Input: part model. Units: mm. Frame: model coordinates. A direction names the side the tool comes from. Coordinates: 2 decimals unless noted, no trailing zeros. Loops run counter-clockwise (first coordinate to the right, second up) from the corner with the lowest first, then second, coordinate; pieces in that order, holes last. Notation, with made-up numbers: (17, 35) - (74, 35) arc R30 ccw to (74, 68) - close; hole circle Ø2 at (21.25, 17). An arc over 180 degrees is marked (long way). Answer as CSV lines item,"result". Start each with the question number.
```python
from build123d import *

# Parameters (mm, degrees)
SM_START               = -47.5
SM_BASE_FLANGE_1_DEPTH = 95
CUT_EXTRUDE_1_DEPTH    = 278.911623222
FILLET_1_R             = 10


# Read off the part's stored shape, not the designer's step: 基体-法兰1
with BuildPart() as part:
    # 基体-法兰1 outline → 基体-法兰1 (new body)
    with BuildSketch(Plane(origin=(0, 0, 0), x_dir=(0, 0, -1), z_dir=(1, 0, 0)).offset(SM_START)):
        with BuildLine():
            Line((20.994484106, 56.207042593), (-70.293536893, 90.304992202))
            Line((-70.293536893, 90.304992202), (-73.092801441, 82.810719856))
            Line((-73.092801441, 82.810719856), (18.195219559, 48.712770248))
            ThreePointArc((18.195219559, 48.712770248), (51.999935218, -0.082081346), (18.041344088, -48.769969279))
            Line((18.041344088, -48.769969279), (-51.521246849, -74.503072197))
            ThreePointArc((-51.521246849, -74.503072197), (-52.886976122, -74.874788174), (-54.296838247, -75))
            Line((-54.296838247, -75), (-212, -75))
            Line((-212, -75), (-212, -83))
            Line((-212, -83), (-54.296838247, -83))
            ThreePointArc((-54.296838247, -83), (-51.477113996, -82.749576348), (-48.74565545, -82.006144394))
            Line((-48.74565545, -82.006144394), (20.816935486, -56.273041476))
            ThreePointArc((20.816935486, -56.273041476), (59.999925251, -0.094709246), (20.994484106, 56.207042593))
        make_face()
    extrude(amount=SM_BASE_FLANGE_1_DEPTH)

    # 草图6 → 切除-拉伸1 (cut, through all)
    with BuildSketch(Plane.XZ.offset(83)):
        with BuildLine():
            Line((-25, 162), (-25, 212))
            Line((-25, 212), (25, 212))
            Line((25, 212), (25, 162))
            ThreePointArc((25, 162), (0, 137), (-25, 162))
        make_face()
    extrude(amount=-CUT_EXTRUDE_1_DEPTH, mode=Mode.SUBTRACT)

    # 圆角1
    fillet_1_edges = [part.edges().sort_by_distance(p)[0] for p in [
        (-25, -79, 212),
        (25, -79, 212),
    ]]
    fillet(fillet_1_edges, radius=FILLET_1_R)


solid = part.part
```
Item 1: Draft query along Y for faces 1 (the cylindrical face through (-0.66, -1.12, -59.99)), 2 (the cylindrical face through (0.55, -79.056, 137.006)), 3 (the flat face through (-0.665, -61.456, 16.253)), 4 (the flat face through (-0.665, 73.017, 24.011)). Return one class per face: pulls with the +Y half, pulls with the -Y half, needs draft (parallel to the pull), parting line crosses it, or undercut.
Item 2: Set-up query: faces 5 (the cylindrical face through (-28.01, -78.94, 209.15)), 6 (the flat face through (-0.66, 66, 28.09)), 7 (the flat face through (47.5, -67, 26)). Return all of +Z, -Z, +X, -X, +Y, -Y with unobstructed straight access to the full face (end or side cutting, diameter ignored); none if empty.
Item 3: Section query B-B, the plane z = 119. Output: boundary loops of the cut face in (x, y).
Item 4: Material intervals for probe 1 along Y at (x, z) = (32, 77); probe 2 along Y at (x, z) = (0.5, 0); probe 3 along Y at (x, z) = (-28, -27), sorted ascending.
Item 5: Section query C-C, the plane y = 19. Output: boundary loops of the cut face in (x, z), and give its area (3 significant figures).
Item 6: Section query A-A, the plane x = 0. Output: boundary loops of the cut face in (y, z) (3 decimals).
Item 7: Contact query for flat-ended pins moving along their axis: P1, Ø6, axis at x = 21, z = 141, coming from the +Y side; P2, Ø5, axis at x = 21.5, y = 21.5, coming from the -Z side; P3, Ø2, axis at x = 24.5, y = -36, coming from the +Z side. Output: stop coordinate, or through.
Response values:
1,face 1,"parting line crosses it"
1,face 2,"needs draft"
1,face 3,"undercut"
1,face 4,"pulls with the +Y half"
2,face 5,"+Z, +Y, -Y"
2,face 6,"+Z, +X, -X"
2,face 7,"+Z, -Z, +X, +Y, -Y"
3,outline,"(-47.5, -83) - (47.5, -83) - (47.5, -75) - (-47.5, -75) - close"
4,probe 1,"y = -83 to -75"
4,probe 2,"y = -63.97 to -55.44, 55.51 to 64.05"
4,probe 3,"y = -53.58 to -44.44, 44.44 to 53.58"
5,outline,"(-47.5, -56.91) - (47.5, -56.91) - (47.5, -48.4) - (-47.5, -48.4) - close"
5,area,"808 mm²"
6,outline,"(-83, 54.297) arc R16 ccw to (-82.006, 48.746) - (-56.273, -20.817) arc R60 ccw to (56.207, -20.994) - (90.305, 70.294) - (82.811, 73.093) - (48.713, -18.195) arc R52 cw to (-48.77, -18.041) - (-74.503, 51.521) arc R8 cw to (-75, 54.297) - (-75, 137) - (-83, 137) - close"
7,P1,"stops at y = -75"
7,P2,"stops at z = -56.91"
7,P3,"stops at z = -36.54"
